```python
from build123d import *

# Parameters (mm, degrees)
F0_R     = 1.5
F1_DEPTH = 3.33
F3_R     = 1.5
F4_DEPTH = 3.33
F2_R     = 1.5
F5_DEPTH = 3.33
F6_SIZE  = 3
F7_R     = 10
F8_SIZE  = 3
F9_R     = 10


with BuildPart() as f1:
    # F0 (on Top) → F1 (new body)
    with BuildSketch(Plane.XY):
        with BuildLine():
            ThreePointArc((-5, -35), (0, -40), (5, -35))
            Line((5, -35), (5, 35))
            ThreePointArc((5, 35), (0, 40), (-5, 35))
            Line((-5, 35), (-5, -35))
        make_face()
        with Locations((0, -35)):
            Circle(F0_R, mode=Mode.SUBTRACT)
        with Locations((0, 35)):
            Circle(F0_R, mode=Mode.SUBTRACT)
    extrude(amount=F1_DEPTH)

    # F3 (on face) → F4 (join)
    with BuildSketch(Plane(origin=(0, 0, 0), x_dir=(1, 0, 0), z_dir=(0, 0, -1))):
        with BuildLine():
            Line((5, -35), (5, -13.4968720376))
            Line((5, -13.4968720376), (-5, -13.4968720376))
            Line((-5, -13.4968720376), (-5, -35))
            ThreePointArc((-5, -35), (0, -40), (5, -35))
        make_face()
        with Locations((0, -35)):
            Circle(F3_R, mode=Mode.SUBTRACT)
    extrude(amount=F4_DEPTH)

    # F2 (on face) → F5 (join)
    with BuildSketch(Plane.XY.offset(3.33)):
        with BuildLine():
            Line((-5, 35), (-5, 13.5650867596))
            Line((-5, 13.5650867596), (5, 13.5650867596))
            Line((5, 13.5650867596), (5, 35))
            ThreePointArc((5, 35), (0, 40), (-5, 35))
        make_face()
        with Locations((0, 35)):
            Circle(F2_R, mode=Mode.SUBTRACT)
    extrude(amount=F5_DEPTH)

    # F6
    f6_edges = [f1.edges().sort_by_distance(p)[0] for p in [
        (0, 13.565087, 6.66),
    ]]
    chamfer(f6_edges, length=F6_SIZE)

    # F7
    f7_edges = [f1.edges().sort_by_distance(p)[0] for p in [
        (0, 16.565087, 6.66),
    ]]
    fillet(f7_edges, radius=F7_R)

    # F8
    f8_edges = [f1.edges().sort_by_distance(p)[0] for p in [
        (0, 13.496872, -3.33),
    ]]
    chamfer(f8_edges, length=F8_SIZE)

    # F9
    f9_edges = [f1.edges().sort_by_distance(p)[0] for p in [
        (0, 16.496872, -3.33),
    ]]
    fillet(f9_edges, radius=F9_R)


solid = f1.part
```
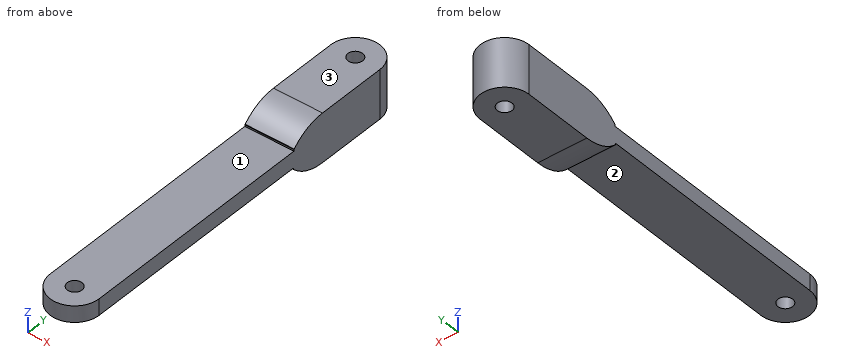
Could you check a few things on this model? Use its own coordinates, in mm. Face numbers are marked on the shaded views. A direction names the side the tool comes from. Coordinates: 2 decimals unless noted, no trailing zeros. Loops run counter-clockwise (first coordinate to the right, second up) from the corner with the lowest first, then second, coordinate; pieces in that order, holes last.
1) Imagine slicing it at A-A (x = 0). List the corners of the cut face in (y, z) for me, and give its area (3 significant figures).
Reported:
outline: (-40, 0) - (-36.5, 0) - (-36.5, 3.33) - (-40, 3.33) - close; (-33.5, 0) - (13.5, 0) - (13.5, -0.33) - (13.57, -0.4) arc R10 ccw to (20.64, -3.33) - (33.5, -3.33) - (33.5, 6.66) - (20.71, 6.66) arc R10 ccw to (13.64, 3.73) - (13.57, 3.66) - (13.57, 3.33) - (-33.5, 3.33) - close; (36.5, -3.33) - (40, -3.33) - (40, 6.66) - (36.5, 6.66) - close
area: 389 mm2
2) Imagine slicing it at D-D (x = -4). List the corners of the cut face in (y, z) for me.
Reported:
outline: (-38, 0) - (13.5, 0) - (13.5, -0.33) - (13.57, -0.4) arc R10 ccw to (20.64, -3.33) - (38, -3.33) - (38, 6.66) - (20.71, 6.66) arc R10 ccw to (13.64, 3.73) - (13.57, 3.66) - (13.57, 3.33) - (-38, 3.33) - close
3) Which directions (+Z, -Z, +X, -X, +Y, -Y) give clear straight access to the entire face, cutting with the end or side of a thin tool? Please do the marked faces 1, 2 and 3.
Reported:
face 1: +Z, +X, -X, -Y
face 2: -Z, +X, -X, -Y
face 3: +Z, +X, -X, +Y, -Y
4) Imagine slicing it at B-B (z = -1.25). List the corners of the cut face in (x, y) for me, and give its area (3 significant figures).
Reported:
outline: (-5, 14.53) - (5, 14.53) - (5, 35) arc R5 ccw to (-5, 35) - close; hole circle Ø3 at (0, 35)
area: 237 mm2
5) Please list where these lines run through material, in increasing order: line 1 along Y through (x, z) = (0, 2.75); line 2 along X through (y, z) = (35, 0.25); line 3 along Z through (x, y) = (4.75, -33).
Reported:
line 1: y = -40 to -36.5, -33.5 to 33.5, 36.5 to 40
line 2: x = -5 to -1.5, 1.5 to 5
line 3: z = 0 to 3.33
6) Will these pins go through, and if not, where does the flat tip stop? pin 1 Ø3 at (x, y) = (1.5, -18) entering from +Z; pin 2 Ø4 at (x, y) = (0, -35) entering from -Z.
Reported:
pin 1: stops at z = 3.33
pin 2: stops at z = 0
7) Imagine slicing it at C-C (y = 0.5). List the corners of the cut face in (x, z) for me.
Reported:
outline: (-5, 0) - (5, 0) - (5, 3.33) - (-5, 3.33) - close
